Answer from the drawing. Dimensions are ordinates in mm from the lowest x, y and z of the part. Give positions to 0.01 mm unless a question says otherwise; leave off trailing zeros. Write each loop counter-clockwise with the first axis right and the second up, starting at its lowest first coordinate (ties: lowest second). Pieces come first, ordered by that corner, then holes. Notation, with made-up numbers: (73.25, -25) -> (97.25, -25) arc R16 cw to (97.25, 1) -> close; hole circle Ø1 at (-7, 74.5). An arc over 180 degrees is marked (long way). Use a Markdown table: item, result. Add a question column.
Q1. Consider line 1 (Z direction, x = 18.35, y = 2.45); line 2 (X direction, y = 0.85, z = 4). Determine where each line is inside the solid, lowest interval first.
Q2. Section A-A, the plane z = 154 is taken. Give the vertices of the cut face in (x, y), plus the area to 3 significant figures.
Q3. This flat-tipped pin is pushed along its axis until it touches: pin 1 Ø3.5 at (x, z) = (74.35, 4) entering from +Y. Where does it stop, or does it pass through?
Q4. Section B-B, the plane x = 18.35 is taken. Give the vertices of the cut face in (y, z).
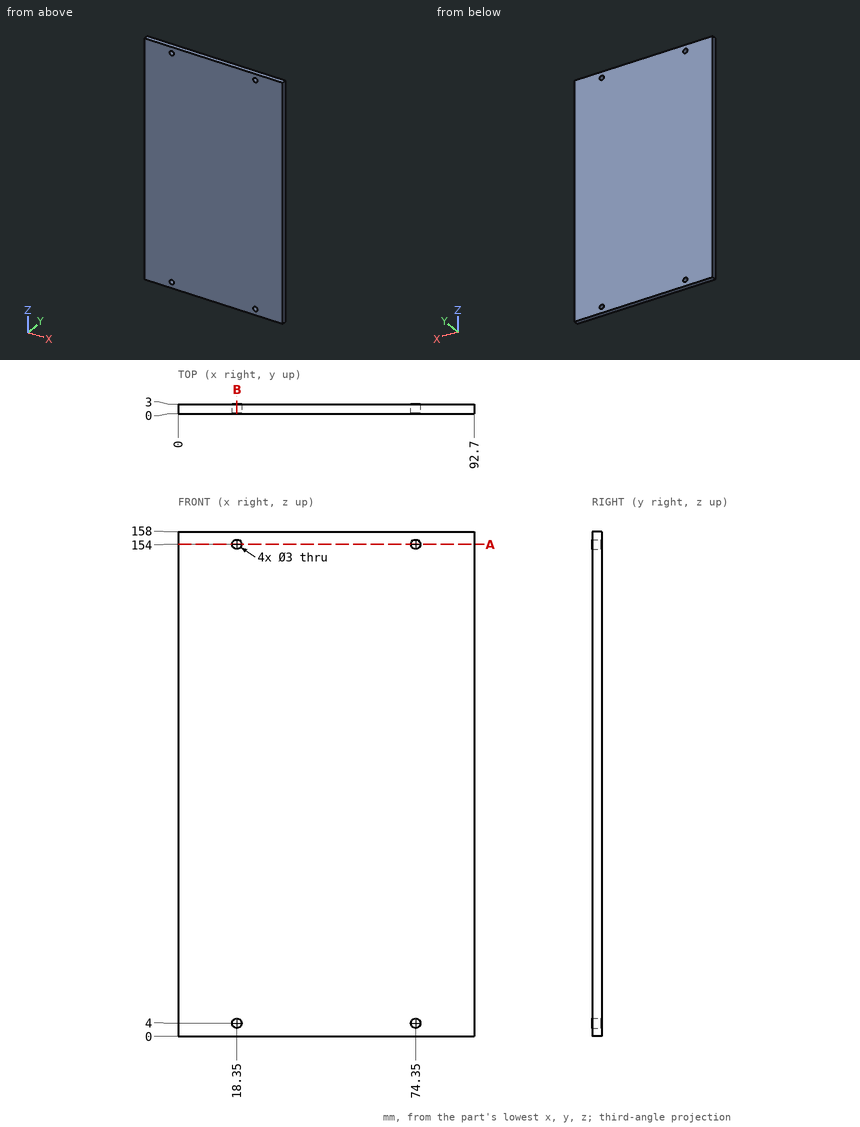
Result set:
| question | item | result |
|---|---|---|
| 1 | line 1 | z = 0 to 2.5, 5.5 to 152.5, 155.5 to 158 |
| 1 | line 2 | x = 0 to 16.85, 19.85 to 72.85, 75.85 to 92.7 |
| 2 | outline | (0, 0) -> (16.85, 0) -> (16.85, 3) -> (0, 3) -> close; (19.85, 0) -> (72.85, 0) -> (72.85, 3) -> (19.85, 3) -> close; (75.85, 0) -> (92.7, 0) -> (92.7, 3) -> (75.85, 3) -> close |
| 2 | area | 260 mm2 |
| 3 | pin 1 | stops at y = 3 |
| 4 | outline | (0, 0) -> (3, 0) -> (3, 2.5) -> (0, 2.5) -> close; (0, 5.5) -> (3, 5.5) -> (3, 152.5) -> (0, 152.5) -> close; (0, 155.5) -> (3, 155.5) -> (3, 158) -> (0, 158) -> close |
